from build123d import *

# Parameters (mm, degrees)
SKETCH1_R           = 9.779
BOSS_EXTRUDE1_DEPTH = 24.384
SKETCH2_W           = 9.652
SKETCH2_H           = 9.652
CUT_EXTRUDE1_DEPTH  = 11.43
CUT_EXTRUDE2_DEPTH  = 12.954
CIRPATTERN1_COUNT   = 2
CIRPATTERN1_ANGLE   = 30
CHAMFER1_SIZE       = 0.5842


with BuildPart() as part:
    # Sketch1 → Boss-Extrude1 (new body)
    with BuildSketch(Plane(origin=(0, 0, 0), x_dir=(1, 0, 0), z_dir=(0, 1, 0))):
        with Locations(Location((0, 0, 0), (0, 0, 90))):
            Circle(SKETCH1_R)
    extrude(amount=BOSS_EXTRUDE1_DEPTH)

    # Sketch2 → Cut-Extrude1 (cut)
    with BuildSketch(Plane.XZ):
        Rectangle(SKETCH2_W, SKETCH2_H)
    extrude(amount=-CUT_EXTRUDE1_DEPTH, mode=Mode.SUBTRACT)

    # Sketch3 → Cut-Extrude2 (cut)
    with BuildSketch(Plane(origin=(0, 24.384, 0), x_dir=(1, 0, 0), z_dir=(0, 1, 0))):
        Polygon((8.30021841, 0), (4.150109205, 7.1882), (-4.150109205, 7.1882), (-8.30021841, 0), (-4.150109205, -7.1882), (4.150109205, -7.1882), align=None)
    cut_extrude2 = extrude(amount=-CUT_EXTRUDE2_DEPTH, mode=Mode.SUBTRACT)

    # CirPattern1: Cut-Extrude2 ×2 about axis
    cirpattern1_axis = Axis((0, 0, 0), (0, 1, 0))
    for i in range(1, CIRPATTERN1_COUNT):
        add(cut_extrude2.rotate(cirpattern1_axis, i * CIRPATTERN1_ANGLE / (CIRPATTERN1_COUNT - 1)), mode=Mode.SUBTRACT)

    # Chamfer1
    chamfer1_edges = [part.edges().sort_by_distance(p)[0] for p in [
        (4.70611841, 24.384, 6.225163807),
        (7.744209205, 24.384, -0.963036193),
        (3.038090795, 24.384, -7.1882),
        (-4.70611841, 24.384, -6.225163807),
        (-7.744209205, 24.384, 0.963036193),
        (-3.038090795, 24.384, 7.1882),
        (7.744209205, 24.384, 0.963036193),
        (3.038090795, 24.384, 7.1882),
        (-4.70611841, 24.384, 6.225163807),
        (-7.744209205, 24.384, -0.963036193),
        (-3.038090795, 24.384, -7.1882),
        (4.70611841, 24.384, -6.225163807),
        (7.1882, 24.384, -3.038090795),
        (6.225163807, 24.384, -4.70611841),
        (0.963036193, 24.384, -7.744209205),
        (-0.963036193, 24.384, -7.744209205),
        (-6.225163807, 24.384, -4.70611841),
        (-7.1882, 24.384, -3.038090795),
        (-7.1882, 24.384, 3.038090795),
        (-6.225163807, 24.384, 4.70611841),
        (-0.963036193, 24.384, 7.744209205),
        (0.963036193, 24.384, 7.744209205),
        (6.225163807, 24.384, 4.70611841),
        (7.1882, 24.384, 3.038090795),
    ]]
    chamfer(chamfer1_edges, length=CHAMFER1_SIZE)


solid = part.part
The listing builds one solid part. Answer for the finished solid, in the listing's coordinates (mm). A direction names the side the tool comes from. Give positions to 0.01 mm unless a question says otherwise; leave off trailing zeros. Order: outer loops, then holes, each group sorted by start corner. A loop starts at its lowest first (then second) coordinate and runs counter-clockwise, first axis right, second up. Notation, with made-up numbers: (72.25, 65) -> (115.25, 65) arc R17 ccw to (115.25, 80) -> close; hole circle Ø2 at (48, -32.5). An arc over 180 degrees is marked (long way). Put each result on its own line as item: value.
Item 1: A cutting plane is placed at D-D on z = -6.5. Give the vertices of the cut face in (x, y).
Established:
outline: (-7.31, 0) -> (7.31, 0) -> (7.31, 24.38) -> (5.22, 24.38) -> (4.55, 23.8) -> (4.55, 11.43) -> (-4.55, 11.43) -> (-4.55, 23.8) -> (-5.22, 24.38) -> (-7.31, 24.38) -> close
Item 2: A cutting plane is placed at B-B on y = 4. Give the vertices of the cut face in (x, z), plus the area to 3 significant figures.
Established:
outline: circle Ø19.56 at (0, 0); hole (-4.83, -4.83) -> (4.83, -4.83) -> (4.83, 4.83) -> (-4.83, 4.83) -> close
area: 207 mm^2
Item 3: Given P1, Ø1.1, axis at x = -3, y = 18, coming from the -Z side; P2, Ø10, axis at y = 3, z = -4, coming from the -X side; P3, Ø5, axis at x = 3.5, y = 3.5, coming from the -Z side; P4, Ø1.5, axis at x = 1, z = -2.5, coming from the -Y side, each flat-ended and moving along its own axis, determine where each tip first touches the part or whether it passes through.
Established:
P1: stops at z = -9.47
P2: stops at x = -9.78
P3: stops at z = -9.73
P4: passes through
Item 4: A cutting plane is placed at A-A on x = -2.75. Give the vertices of the cut face in (y, z).
Established:
outline: (0, -9.38) -> (24.38, -9.38) -> (24.38, -7.77) -> (23.8, -7.19) -> (11.43, -7.19) -> (11.43, -4.83) -> (0, -4.83) -> close; (0, 4.83) -> (11.43, 4.83) -> (11.43, 7.19) -> (23.8, 7.19) -> (24.38, 7.77) -> (24.38, 9.38) -> (0, 9.38) -> close
Item 5: For faces 1 (the face through (0, 6, -4.826)), 2 (the face through (0.98, 24.09, -8.07)), determine the directions among +Z, -Z, +X, -X, +Y, -Y from which every point of the face is accessible in a straight line to the end or side of a thin tool.
Established:
face 1: +Y, -Y
face 2: +Y
Item 6: A cutting plane is placed at C-C on z = -0.75. Give the vertices of the cut face in (x, y), plus the area to 3 significant figures.
Established:
outline: (-9.75, 0) -> (-4.83, 0) -> (-4.83, 11.43) -> (-7.87, 11.43) -> (-7.87, 23.8) -> (-8.54, 24.38) -> (-9.75, 24.38) -> close; (4.83, 0) -> (9.75, 0) -> (9.75, 24.38) -> (8.54, 24.38) -> (7.87, 23.8) -> (7.87, 11.43) -> (4.83, 11.43) -> close
area: 161 mm^2
Item 7: Straight lines are drawn through the part: line 1 (Z direction, x = 0.25, y = 1.75); line 2 (X direction, y = 19, z = 6.5); line 3 (Y direction, x = -1.5, z = 6.75). For each, find the intervals that lie inside material, in ascending order.
Established:
line 1: z = -9.78 to -4.83, 4.83 to 9.78
line 2: x = -7.31 to -4.55, 4.55 to 7.31
line 3: y = 0 to 11.43
